Work out the finished part from the listing and answer in its coordinate system (mm). A direction names the side the tool comes from. Round coordinates to 2 decimals unless told otherwise and drop trailing zeros. Write each loop counter-clockwise with the first axis right and the second up, starting at its lowest first coordinate (ties: lowest second). Pieces come first, ordered by that corner, then holes.
1. Find section B-B (x = -17.5). Write down the section's boundary in (y, z).
2. Straight lines are drawn through the part: probe 1 along Z at (x, y) = (30, -6); probe 2 along Y at (x, z) = (17.5, -7.5); probe 3 along Y at (x, z) = (-11.5, 9). For each, find the intervals that lie inside material, in ascending order.
3. Find section C-C (y = 15.5). Write down the section's boundary in (x, z), and give its area (3 significant figures).
4. Find section A-A (y = 42.5). Write down the section's boundary in (x, z).
5. Flat-ended cylindrical pins translate along their axes: pin 1 Ø3 at (x, z) = (-12, 2.5) entering from +Y; pin 2 Ø12 at (x, y) = (-11.5, -2.5) entering from -Z; pin 3 Ø12 at (y, z) = (18, -8) entering from +X. Find the tip coordinate at first contact, or state that the pin passes through.
6. A tool of negligible diameter and unlimited length cuts with its end or side. For faces 1 (the face through (0.784, 37.073, 1.012)), 2 (the face through (-2.716, 23.704, -4.468)), 3 (the face through (3.642, 10.382, -3.542)), 4 (the face through (3.415, 29.168, 3.769)), from which of +Z, -Z, +X, -X, +Y, -Y can it reach the whole face along a straight path? Write none if from no direction.
7. Determine the mould class of faces 5 (the face through (2, 47.189, 1)), 6 (the face through (1.29, 26.66, -1.29)), 7 (the face through (11.727, 31.403, -11.626)), 8 (the face through (13.251, 38.461, -8.446)) for opening direction Z: pulls with the +Z half, pulls with the -Z half, needs draft (parallel to the pull), parting line crosses it, or undercut.
```python
from build123d import *

# Parameters (mm, degrees)
SKETCH1_W                 = 81.28
SKETCH1_H                 = 25.4
BOSS_EXTRUDE1_DEPTH       = 10.16
BOSS_EXTRUDE2_DEPTH       = 25.4
BOSS_EXTRUDE3_DEPTH       = 10.16
BOSS_EXTRUDE4_DEPTH       = 3.81
BOSS_EXTRUDE5_DEPTH       = 5.08
F_8_32_TAPPED_HOLE2_D     = 3.4544
F_8_32_TAPPED_HOLE2_DEPTH = 7.62
F_8_32_TAPPED_HOLE2_TIP   = 1.037806461


with BuildPart() as part:
    # Sketch1 → Boss-Extrude1 (new body)
    # profile 1 of 2: a face of its own
    with BuildSketch(Plane(origin=(0, 0, 0), x_dir=(1, 0, 0), z_dir=(0, 1, 0))):
        Rectangle(SKETCH1_W, SKETCH1_H)
        Polygon((7.184204897, 0), (0, 7.184204897), (-7.184204897, 0), (0, -7.184204897), align=None, mode=Mode.SUBTRACT)
    # profile 2 of 2: a face of its own
    with BuildSketch(Plane(origin=(0, 0, 0), x_dir=(1, 0, 0), z_dir=(0, 1, 0))):
        Polygon((0, -7.184204897), (7.184204897, 0), (0, 7.184204897), (-7.184204897, 0), align=None)
    extrude(amount=-BOSS_EXTRUDE1_DEPTH)

    # Sketch1<3> → Boss-Extrude2 (add)
    with BuildSketch(Plane(origin=(0, 0, 0), x_dir=(1, 0, 0), z_dir=(0, 1, 0))):
        Polygon((0, -7.184204897), (7.184204897, 0), (0, 7.184204897), (-7.184204897, 0), align=None)
    extrude(amount=BOSS_EXTRUDE2_DEPTH)

    # Sketch3 → Boss-Extrude3 (add)
    with BuildSketch(Plane(origin=(3.592102448, 0, 3.592102448), x_dir=(0.7071067811865472, 0, -0.7071067811865479), z_dir=(0.7071067811865479, 0, 0.7071067811865472))):
        with BuildLine():
            ThreePointArc((0, 25.4), (-11.791936413, 33.279120011), (-9.025157402, 47.188657402))
            Line((-9.025157402, 47.188657402), (-15.392758886, 47.188657402))
            ThreePointArc((-15.392758886, 47.188657402), (0, 20.32), (15.392758886, 47.188657402))
            Line((15.392758886, 47.188657402), (9.025157402, 47.188657402))
            ThreePointArc((9.025157402, 47.188657402), (11.791936413, 33.279120011), (0, 25.4))
        make_face()
    extrude(amount=-BOSS_EXTRUDE3_DEPTH)

    # Sketch3<3> → Boss-Extrude4 (add)
    with BuildSketch(Plane(origin=(3.592102448, 0, 3.592102448), x_dir=(0.7071067811865472, 0, -0.7071067811865479), z_dir=(0.7071067811865479, 0, 0.7071067811865472))):
        with BuildLine():
            Line((15.392758886, 47.188657402), (-15.392758886, 47.188657402))
            ThreePointArc((-15.392758886, 47.188657402), (0, 20.32), (15.392758886, 47.188657402))
        make_face()
    extrude(amount=-BOSS_EXTRUDE4_DEPTH)

    # Sketch3<4> → Boss-Extrude5 (add)
    with BuildSketch(Plane(origin=(3.592102448, 0, 3.592102448), x_dir=(0.7071067811865472, 0, -0.7071067811865479), z_dir=(0.7071067811865479, 0, 0.7071067811865472))):
        with BuildLine():
            Line((-7.116675918, 47.188657402), (-9.025157402, 47.188657402))
            ThreePointArc((-9.025157402, 47.188657402), (-11.791936413, 33.279120011), (0, 25.4))
            ThreePointArc((0, 25.4), (11.791936413, 33.279120011), (9.025157402, 47.188657402))
            Line((9.025157402, 47.188657402), (7.116675918, 47.188657402))
            ThreePointArc((7.116675918, 47.188657402), (0, 26.67), (-7.116675918, 47.188657402))
        make_face()
    extrude(amount=-BOSS_EXTRUDE5_DEPTH)

    # #8-32 Tapped Hole2
    with Locations(Plane(origin=(-3.592102448, 0, -3.592102448), x_dir=(-0.7071067811865472, 0, 0.7071067811865479), z_dir=(-0.7071067811865479, 0, -0.7071067811865472))):
        with Locations((15.3035, 38.1635), (-15.3035, 38.1635)):
            Hole(F_8_32_TAPPED_HOLE2_D / 2, depth=F_8_32_TAPPED_HOLE2_DEPTH)
            with Locations((0, 0, -(F_8_32_TAPPED_HOLE2_DEPTH + F_8_32_TAPPED_HOLE2_TIP / 2))):  # 118° drill point
                Cone(0, F_8_32_TAPPED_HOLE2_D / 2, F_8_32_TAPPED_HOLE2_TIP, mode=Mode.SUBTRACT)


solid = part.part
```
Worked answers:
1. outline: (-10.16, -12.7) - (0, -12.7) - (0, 12.7) - (-10.16, 12.7) - close
2. probe 1: z = -12.7 to 12.7
2. probe 2: y = -10.16 to 0
2. probe 3: y = -10.16 to 0, 27.76 to 36.64, 39.69 to 47.19
3. outline: (-7.18, 0) - (0, -7.18) - (7.18, 0) - (0, 7.18) - close
3. area: 103 mm2
4. outline: (-15.83, 8.65) - (-12.08, 4.9) - (-8.49, 8.49) - (-7.53, 7.53) - (-6.63, 8.42) - (8.42, -6.63) - (7.53, -7.53) - (8.49, -8.49) - (4.9, -12.08) - (8.65, -15.83) - (15.83, -8.65) - (-8.65, 15.83) - close
5. pin 1: stops at y = 0
5. pin 2: stops at z = -12.7
5. pin 3: stops at x = 8.79
6. face 1: none
6. face 2: -Z, -X, +Y
6. face 3: -Z, +X
6. face 4: +Z, +X, +Y
7. face 5: needs draft
7. face 6: undercut
7. face 7: pulls with the -Z half
7. face 8: undercut
